from build123d import *

# Parameters (mm, degrees)
F0_W     = 124.630935
F0_H     = 75.701751
F1_DEPTH = 12.7
F2_W     = 39.33452
F2_H     = 16.389386
F3_DEPTH = 25.4
F4_W     = 26.818996
F4_H     = 26.818994
F5_DEPTH = 6.35
F6_R     = 1.800148
F7_DEPTH = 2.54


with BuildPart() as f1:
    # F0 (on Top) → F1 (new body)
    with BuildSketch(Plane.XY):
        with Locations((4.154365, -3.461972)):
            Rectangle(F0_W, F0_H)
    extrude(amount=F1_DEPTH)

    # F2 (on face) → F3 (join)
    with BuildSketch(Plane.XY.offset(12.7)):
        with Locations((42.6124, -2.383911)):
            Rectangle(F2_W, F2_H)
    extrude(amount=F3_DEPTH)

    # F4 (on face) → F5 (join)
    with BuildSketch(Plane.XY.offset(12.7)):
        with Locations((-34.566705, -1.042961)):
            Rectangle(F4_W, F4_H)
    extrude(amount=F5_DEPTH)

    # F6 (on face) → F7 (join)
    with BuildSketch(Plane.XZ.offset(10.578604)):
        with Locations((41.615058, 25.010286)):
            Circle(F6_R)
    extrude(amount=F7_DEPTH)


solid = f1.part
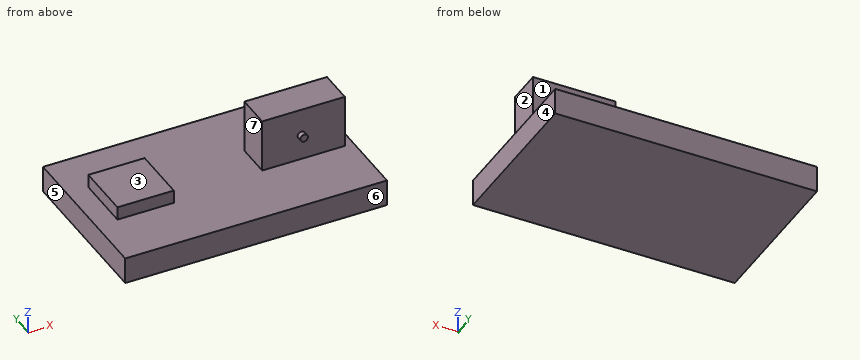
The listing builds one solid part. Answer for the finished solid, in the listing's coordinates (mm). Face numbers are marked on the shaded views. A direction names the side the tool comes from. Give positions to 0.01 mm unless a question says otherwise; leave off trailing zeros. Loops run counter-clockwise (first coordinate to the right, second up) from the corner with the lowest first, then second, coordinate; pieces in that order, holes last.
Item 1: A cutting plane is placed at C-C (z = 35.5). Give the vertices of the cut face in (x, y).
Derived:
outline: (22.95, -10.58) - (62.28, -10.58) - (62.28, 5.81) - (22.95, 5.81) - close
Item 2: Find the intervals of material crossed by line 1 along Z through (x, y) = (-11, -20); line 2 along Y through (x, z) = (49.5, 24); line 3 along X through (y, z) = (-5.5, 27), in increasing order.
Derived:
line 1: z = 0 to 12.7
line 2: y = -10.58 to 5.81
line 3: x = 22.95 to 62.28
Item 3: Each of these flat-tipped pins is pushed along its axis until it touches: pin 1 Ø7.5 at (x, z) = (35.5, 19.5) entering from +Y; pin 2 Ø13 at (y, z) = (-0.5, 25) entering from -X; pin 3 Ø6 at (x, y) = (14, -29.5) entering from +Z. Where does it stop, or does it pass through?
Derived:
pin 1: stops at y = 5.81
pin 2: stops at x = -47.98
pin 3: stops at z = 12.7
Item 4: Determine the mould class of the marked faces 5, 6 and 7 for opening direction X: +X half, -X half, draft (parallel to the pull), parting line (faces both ways), or undercut.
Derived:
face 5: -X half
face 6: draft
face 7: undercut
Item 5: A cutting plane is placed at A-A (y = -9). Give the vertices of the cut face in (x, z), then the cut area to 3 significant figures.
Derived:
outline: (-58.16, 0) - (66.47, 0) - (66.47, 12.7) - (62.28, 12.7) - (62.28, 38.1) - (22.95, 38.1) - (22.95, 12.7) - (-21.16, 12.7) - (-21.16, 19.05) - (-47.98, 19.05) - (-47.98, 12.7) - (-58.16, 12.7) - close
area: 2,750 mm2
Item 6: A cutting plane is placed at D-D (x = -22.5). Give the vertices of the cut face in (y, z).
Derived:
outline: (-41.31, 0) - (34.39, 0) - (34.39, 12.7) - (12.37, 12.7) - (12.37, 19.05) - (-14.45, 19.05) - (-14.45, 12.7) - (-41.31, 12.7) - close
Item 7: A tool of negligible diameter and unlimited length cuts with its end or side. For the marked faces 1, 2, 3 and 4, from which of +Z, -Z, +X, -X, +Y, -Y can it reach the whole face along a straight path? Write none if from no direction.
Derived:
face 1: +Z, +X, +Y
face 2: +Z, +X, +Y, -Y
face 3: +Z, -X, +Y, -Y
face 4: +Z, -Z, +X, +Y, -Y
Item 8: A cutting plane is placed at B-B (x = 36.5). Give the vertices of the cut face in (y, z).
Derived:
outline: (-41.31, 0) - (34.39, 0) - (34.39, 12.7) - (5.81, 12.7) - (5.81, 38.1) - (-10.58, 38.1) - (-10.58, 12.7) - (-41.31, 12.7) - close
